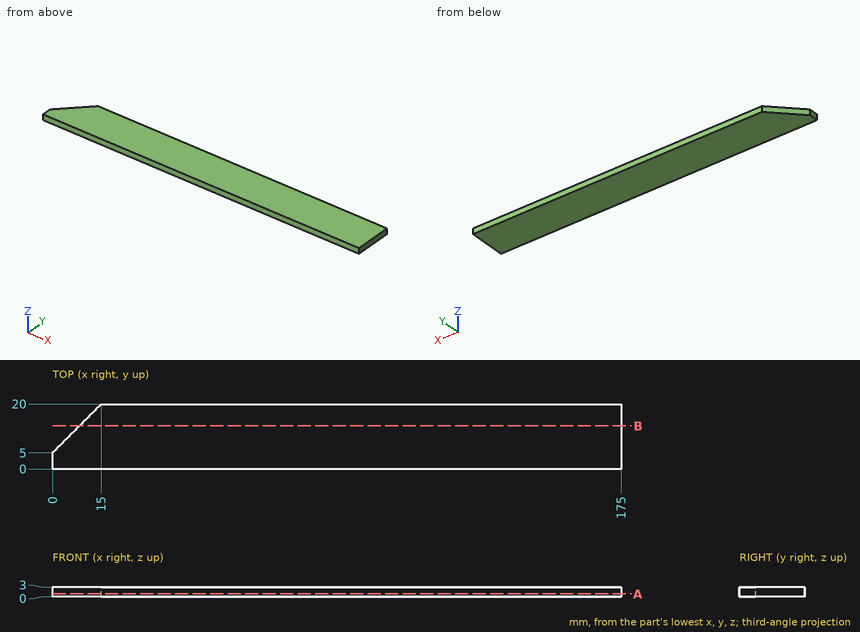
For this review, use the dimensioned drawing (mm, ordinates from the lowest corner) and the shaded views. Round coordinates to 2 decimals unless told otherwise and drop trailing zeros. Write each loop counter-clockwise with the first axis right and the second up, starting at its lowest first coordinate (ties: lowest second). Pieces come first, ordered by that corner, then holes. Notation, with made-up numbers: M -36,-15.5 L 4,-15.5 A17 cw 4,12.5 Z; hole C 25,75 d2. An arc over 180 degrees is marked long. Answer as CSV lines item,"result". Start each with the question number.
Q1. Consider section B-B, the plane y = 13.25. Give the boundary of the cut face in (x, z).
Q2. Wall thickness on line 1 along X through (y, z) = (10.25, 1.4); line 2 along Y through (x, z) = (7.5, 1.3); line 3 along X through (y, z) = (9, 0.3): over which ranges is each line inside the solid? List them lowest first.
Q3. Consider section A-A, the plane z = 0.9. Give the boundary of the cut face in (x, y).
Result set:
1,outline,"M 8.25,0 L 175,0 L 175,3 L 8.25,3 Z"
2,line 1,"x = 5.25 to 175"
2,line 2,"y = 0 to 12.5"
2,line 3,"x = 4 to 175"
3,outline,"M 0,0 L 175,0 L 175,20 L 15,20 L 0,5 Z"
